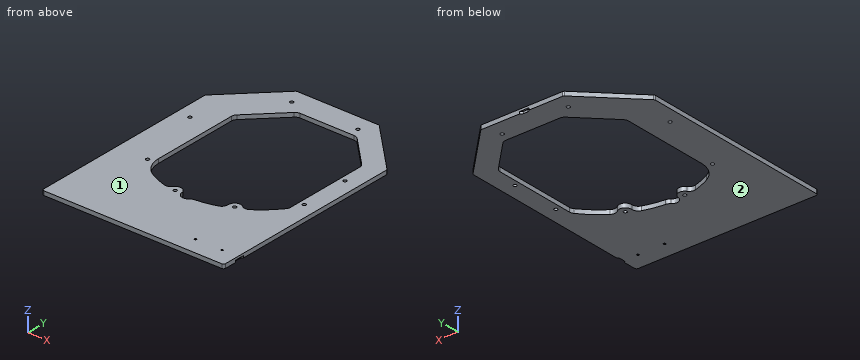
```python
from build123d import *

# Parameters (mm, degrees)
BOSS_EXTRUDE1_DEPTH              = 6.35
F_13_64_0_20313_DIAMETER_HOLE1_D = 5.159502
FILLET1_R                        = 3.175
CUT_EXTRUDE1_DEPTH               = 3.175
F_4_40_TAPPED_HOLE1_AT_2_COUNT   = 2
F_4_40_TAPPED_HOLE1_AT_2_PITCH   = 40.8813


with BuildPart() as part:
    # Sketch1 → Boss-Extrude1 (new body)
    with BuildSketch(Plane.XY):
        Polygon((63.5, 139.7), (139.7, 63.5), (139.7, -234.95), (-139.7, -234.95), (-139.7, 63.5), (-63.5, 139.7), align=None)
        with BuildLine():
            Line((-32.547758941, 98.810192091), (-80.392170491, 50.965780541))
            ThreePointArc((-80.392170491, 50.965780541), (-82.456930947, 47.875648143), (-83.1819784, 44.23058845))
            Line((-83.1819784, 44.23058845), (-83.1819784, -88.9))
            ThreePointArc((-83.1819784, -88.9), (-77.397388735, -109.262606079), (-61.771467321, -123.542934642))
            ThreePointArc((-61.771467321, -123.542934642), (-49.690626762, -128.877509625), (-37.155545476, -133.033966773))
            ThreePointArc((-37.155545476, -133.033966773), (-31.397184902, -132.845734548), (-26.785398712, -129.39239182))
            ThreePointArc((-26.785398712, -129.39239182), (-16.51294166, -125.769298085), (-9.558427406, -134.152907902))
            ThreePointArc((-9.558427406, -134.152907902), (-3.356200416, -142.335772885), (6.691703581, -140.222357584))
            ThreePointArc((6.691703581, -140.222357584), (9.354962656, -138.393777353), (12.476251165, -137.560583133))
            ThreePointArc((12.476251165, -137.560583133), (28.622348201, -135.127095945), (44.368454999, -130.805241011))
            ThreePointArc((44.368454999, -130.805241011), (49.212504081, -127.100822664), (50.816921447, -121.217509676))
            ThreePointArc((50.816921447, -121.217509676), (56.065290503, -112.130581006), (66.483854873, -113.384042964))
            ThreePointArc((66.483854873, -113.384042964), (72.153155683, -115.630496863), (78.02311981, -113.977908606))
            ThreePointArc((78.02311981, -113.977908606), (94.714050954, -100.537651788), (109.125182698, -84.677419518))
            ThreePointArc((109.125182698, -84.677419518), (110.611187219, -81.924253334), (111.125, -78.838134428))
            Line((111.125, -78.838134428), (111.125, 47.718463274))
            ThreePointArc((111.125, 47.718463274), (110.399952547, 51.363522967), (108.335192091, 54.453655364))
            Line((108.335192091, 54.453655364), (63.978655364, 98.810192091))
            ThreePointArc((63.978655364, 98.810192091), (60.888522967, 100.874952547), (57.243463274, 101.6))
            Line((57.243463274, 101.6), (-25.81256685, 101.6))
            ThreePointArc((-25.81256685, 101.6), (-29.457626543, 100.874952547), (-32.547758941, 98.810192091))
        make_face(mode=Mode.SUBTRACT)
    extrude(amount=-BOSS_EXTRUDE1_DEPTH)

    # 13/64 (0.20313) Diameter Hole1 (through all)
    with Locations(Plane(origin=(-107.95, -107.95, 0), x_dir=(1, 0, 0), z_dir=(0, 0, 1))):
        with Locations((158.75, 223.8502), (57.15, 223.8502), (227.0252, 119.0752), (-11.1252, 119.0752), (227.0252, 44.45), (168.275, -12.7), (88.9, -27.0002), (15.875, 9.525)):
            Hole(F_13_64_0_20313_DIAMETER_HOLE1_D / 2)

    # Fillet1
    fillet1_edges = [part.edges().sort_by_distance(p)[0] for p in [
        (139.7, -234.95, -3.175),
        (-139.7, -234.95, -3.175),
        (-139.7, 63.5, -3.175),
        (-63.5, 139.7, -3.175),
        (63.5, 139.7, -3.175),
        (139.7, 63.5, -3.175),
    ]]
    fillet(fillet1_edges, radius=FILLET1_R)

    # Sketch11 → Cut-Extrude1 (cut)
    with BuildSketch(Plane(origin=(0, 0, -6.35), x_dir=(-1, 0, 0), z_dir=(0, 0, -1))):
        with BuildLine():
            Line((-177.07961661, -198.4248), (-142.0622, -198.4248))
            ThreePointArc((-142.0622, -198.4248), (-138.685623698, -199.823423698), (-137.287, -203.2))
            Line((-137.287, -203.2), (-137.287, -209.5246))
            ThreePointArc((-137.287, -209.5246), (-138.685623698, -212.901176302), (-142.0622, -214.2998))
            Line((-142.0622, -214.2998), (-177.07961661, -214.2998))
            Line((-177.07961661, -214.2998), (-177.07961661, -198.4248))
        make_face()
        with BuildLine():
            Line((-4.7498, 156.359665344), (11.1252, 156.359665344))
            Line((11.1252, 156.359665344), (11.1252, 142.0622))
            ThreePointArc((11.1252, 142.0622), (9.726576302, 138.685623698), (6.35, 137.287))
            Line((6.35, 137.287), (0.0254, 137.287))
            ThreePointArc((0.0254, 137.287), (-3.351176302, 138.685623698), (-4.7498, 142.0622))
            Line((-4.7498, 142.0622), (-4.7498, 156.359665344))
        make_face()
    extrude(amount=-CUT_EXTRUDE1_DEPTH, mode=Mode.SUBTRACT)

    # Sketch14 → #4-40 Tapped Hole1 (revolve, cut)
    with BuildSketch(Plane(origin=(115.6843, -209.55, 0), x_dir=(0, -1, 0), z_dir=(1, 0, 0))):
        Polygon((0, 0), (0, 6.35), (1.651, 6.35), (1.1303, 5.8293), (1.1303, 0.3937), (1.524, 0), align=None)
    f_4_40_tapped_hole1 = revolve(axis=Axis((115.6843, -209.55, 6.35), (0, 0, -1)), mode=Mode.SUBTRACT)

    # #4-40 Tapped Hole1 at 2: #4-40 Tapped Hole1 ×2
    with Locations(*[(-i * F_4_40_TAPPED_HOLE1_AT_2_PITCH, 0, 0) for i in range(1, F_4_40_TAPPED_HOLE1_AT_2_COUNT)]):
        add(f_4_40_tapped_hole1, mode=Mode.SUBTRACT)


solid = part.part
```
Source: CAD feature listing. Evaluate the final solid. Frame: model axes, mm. Face numbers are marked on the shaded views. Coordinates: 2 decimals unless noted, no trailing zeros. Loops run counter-clockwise (first coordinate to the right, second up) from the corner with the lowest first, then second, coordinate; pieces in that order, holes last. Notation, with made-up numbers: M 54,42.5 L 78,42.5 A22 ccw 78,69.5 Z; hole C 35.5,22.5 d2. An arc over 180 degrees is marked long. Use a Markdown table: item, result. Add a question column.
Q1. Draft query along Z for the marked faces 1 and 2. Return one class per face: pulls with the +Z half, pulls with the -Z half, needs draft (parallel to the pull), parting line crosses it, or undercut.
Q2. Section query A-A, the plane y = -49. Return loops of the section in (x, z) (3 decimals), and give its area (3 significant figures).
Q3. Material intervals for L1, parallel to X at y = -209.55, z = -3.45; L2, parallel to Y at x = -19.05, z = -3.75; L3, parallel to X at y = -209.55, z = -1.55, sorted ascending.
Q4. Section query B-B, the plane x = 23. Return loops of the section in (y, z).
Q5. First-contact query: pin 1 (2.5 mm diameter, centred on x = 115.68, y = -209.55, fed in from -Z); pin 2 (0.7 mm diameter, centred on x = 138.5, y = -207, fed in from -Z) (3 decimals); pin 3 (3.5 mm diameter, centred on x = -4, z = -5, fed in from +Y). Flat tips, straight axial feed; report the tip coordinate or a pass-through.
Q6. Section query C-C, the plane z = -1.75. State how many separate pieces and enclosed holes the cut face has, and give its area (3 significant figures).
Result:
| question | item | result |
|---|---|---|
| 1 | face 1 | pulls with the +Z half |
| 1 | face 2 | pulls with the -Z half |
| 2 | outline | M -139.7,-6.35 L -83.182,-6.35 L -83.182,0 L -139.7,0 Z; M 111.125,-6.35 L 139.7,-6.35 L 139.7,0 L 111.125,0 Z |
| 2 | area | 540 mm2 |
| 3 | L1 | x = -139.7 to 73.67, 75.93 to 114.55, 116.81 to 137.29 |
| 3 | L2 | y = -234.95 to -137.53, -132.37 to -125.43, 101.6 to 139.7 |
| 3 | L3 | x = -139.7 to 73.67, 75.93 to 114.55, 116.81 to 139.7 |
| 4 | outline | M -234.95,-6.35 L -136.2,-6.35 L -136.2,0 L -234.95,0 Z; M 101.6,-6.35 L 139.7,-6.35 L 139.7,0 L 101.6,0 Z |
| 5 | pin 1 | stops at z = -5.95 |
| 5 | pin 2 | stops at z = -3.175 |
| 5 | pin 3 | stops at y = 137.29 |
| 6 | separate pieces | 1 |
| 6 | enclosed holes | 11 |
| 6 | area | 57,800 mm2 |
